Can you work these out from the model? Positions are in its coordinate system, mm. Coordinates: 2 decimals unless noted, no trailing zeros. Order: outer loops, then holes, each group sorted by start corner. A loop starts at its lowest first (then second) coordinate and runs counter-clockwise, first axis right, second up. Notation, with made-up numbers: (-12.5, 71) -> (44.5, 71) arc R21 cw to (44.5, 78) -> close; hole circle Ø7 at (30.5, 19). An arc over 180 degrees is marked (long way). Write item = value, one per line.
```python
from build123d import *

# Parameters (mm, degrees)
SKETCH_1_W          = 120
SKETCH_1_H          = 15
EXTRUDE_1_DEPTH     = 5
SKETCH_2_R          = 1.6
SKETCH_2_R_2        = 2.25
CUT_EXTRUDE_1_DEPTH = 6
FILLET_1_R          = 5


with BuildPart() as part:
    # Эскиз1 → Бобышка-Вытянуть1 (new body)
    with BuildSketch(Plane(origin=(0, 0, 0), x_dir=(1, 0, 0), z_dir=(0, 1, 0))):
        with Locations((60, 7.5)):
            Rectangle(SKETCH_1_W, SKETCH_1_H)
    extrude(amount=EXTRUDE_1_DEPTH)

    # Эскиз2 → Вырез-Вытянуть1 (cut, through all)
    with BuildSketch(Plane(origin=(0, 5, 0), x_dir=(1, 0, 0), z_dir=(0, 1, 0))):
        with Locations((13.55, 7.5)):
            Circle(SKETCH_2_R)
        with Locations((106.45, 7.5)):
            Circle(SKETCH_2_R)
        with Locations((60, 7.5)):
            Circle(SKETCH_2_R_2)
    extrude(amount=-CUT_EXTRUDE_1_DEPTH, mode=Mode.SUBTRACT)

    # Скругление1
    fillet_1_edges = [part.edges().sort_by_distance(p)[0] for p in [
        (0, 2.5, -15),
        (120, 2.5, -15),
        (120, 2.5, 0),
        (0, 2.5, 0),
    ]]
    fillet(fillet_1_edges, radius=FILLET_1_R)


solid = part.part
```
Item 1: I'm going to push a flat-ended pin straight in: P1, Ø2.5, axis at x = 13.55, z = -7.5, coming from the -Y side. Where does the tip first touch, or does it pass through?
A:
P1 = through
Item 2: I want a section at A-A, the plane x = 14. Please give me the cut outline in (y, z).
A:
outline = (0, -15) -> (5, -15) -> (5, -9.04) -> (0, -9.04) -> close; (0, -5.96) -> (5, -5.96) -> (5, 0) -> (0, 0) -> close
Item 3: If we mould it in two halves opening along X, with no side actions, what happens to faces 1 (the flat face through (120, 2, -7)), 2 (the cylindrical face through (13.2, 2.54, -5.94)), 3 (the cylindrical face through (1, 3, -2))? For each: pulls with the +X half, pulls with the -X half, needs draft (parallel to the pull), parting line crosses it, or undercut.
A:
face_1 = pulls with the +X half
face_2 = undercut
face_3 = pulls with the -X half
Item 4: I want a section at B-B, the plane y = 1.25. Please give me the cut outline in (x, z).
A:
outline = (0, -10) arc R5 ccw to (5, -15) -> (115, -15) arc R5 ccw to (120, -10) -> (120, -5) arc R5 ccw to (115, 0) -> (5, 0) arc R5 ccw to (0, -5) -> close; hole circle Ø3.2 at (13.55, -7.5); hole circle Ø4.5 at (60, -7.5); hole circle Ø3.2 at (106.45, -7.5)
Item 5: I want a section at C-C, the plane x = 106.45. Please give me the cut outline in (y, z), plus the area to 3 significant figures.
A:
outline = (0, -15) -> (5, -15) -> (5, -9.1) -> (0, -9.1) -> close; (0, -5.9) -> (5, -5.9) -> (5, 0) -> (0, 0) -> close
area = 59.0 mm2
Item 6: If I drill on probe 1 along X at (y, z) = (1.1, -7.5); probe 2 along Z at (x, y) = (13.55, 1.35); probe 3 along Z at (x, y) = (60, 1.25), over which ranges is the centre line in solid material (lowest first)?
A:
probe_1 = 0 to 11.95, 15.15 to 57.75, 62.25 to 104.85, 108.05 to 120
probe_2 = -15 to -9.1, -5.9 to 0
probe_3 = -15 to -9.75, -5.25 to 0
